Here's how the part is built. I have some questions about the finished solid (model axes, mm). Face numbers are marked on the shaded views. Round coordinates to 2 decimals unless told otherwise and drop trailing zeros. Loops run counter-clockwise (first coordinate to the right, second up) from the corner with the lowest first, then second, coordinate; pieces in that order, holes last. Notation, with made-up numbers: (32, 27) - (48, 27) arc R24 ccw to (48, 62) - close; hole circle Ø3 at (26.25, -30). An arc over 180 degrees is marked (long way). Answer as a JSON object with one key per item and string values. Group by question number.
1) I want a section at A-A, the plane y = 0. Please give me the cut outline in (x, z) (3 decimals).
2) Will these pins go through, and if not, where does the flat tip stop? P1, Ø4, axis at y = -2.5, z = 18.5, coming from the -X side; P2, Ø6, axis at x = -24.5, z = 106, coming from the -Y side; P3, Ø12, axis at y = -17.5, z = 15, coming from the -X side.
3) I want a section at B-B, the plane z = 23. Please give me the cut outline in (x, y) (3 decimals), then the cut area to 3 significant figures.
4) If we mould it in two halves opening along Y, with no side actions, what happens to the marked faces 1, 2 and 3? For each: pulls with the +Y half, pulls with the -Y half, needs draft (parallel to the pull), parting line crosses it, or undercut.
5) If I drill on line 1 along Y through (x, z) = (0, 42.5) (3 decimals); line 2 along Z through (x, y) = (-20.5, -23); line 3 along X through (y, z) = (-19, 71), over which ranges is the centre line in solid material (lowest first)? Write a range as [from, to].
from build123d import *

# Parameters (mm, degrees)
F0_R     = 38.1
F0_R_2   = 34.925
F1_DEPTH = 127
F2_R     = 34.925
F3_DEPTH = 2.54


# Not quite as in the source:
# - a fillet or chamfer that OpenCascade refuses, or shapes differently, is made with other operations: its cross-section is extruded or revolved along the edge and cut away or added


with BuildPart() as f1:
    # F0 (on Top) → F1 (new body)
    with BuildSketch(Plane.XY):
        Circle(F0_R)
        Circle(F0_R_2, mode=Mode.SUBTRACT)
    extrude(amount=F1_DEPTH)

    # F2 (on Top) → F3 (join)
    with BuildSketch(Plane.XY):
        Circle(F2_R)
    extrude(amount=F3_DEPTH)

    # F4: fillet of radius 5.08 on 1 edges, made by hand

    # F4_s1 → F4_t2 (revolve, cut)
    with BuildSketch(Plane.XZ):
        with BuildLine():
            ThreePointArc((38.1, 122.2907139607), (37.2321134838, 125.1305202921), (34.925, 127))
            Line((34.925, 127), (38.1, 127))
            Line((38.1, 127), (38.1, 122.2907139607))
        make_face()
    revolve(axis=Axis((0, 0, 127), (0, 0, 1)), mode=Mode.SUBTRACT)


solid = f1.part
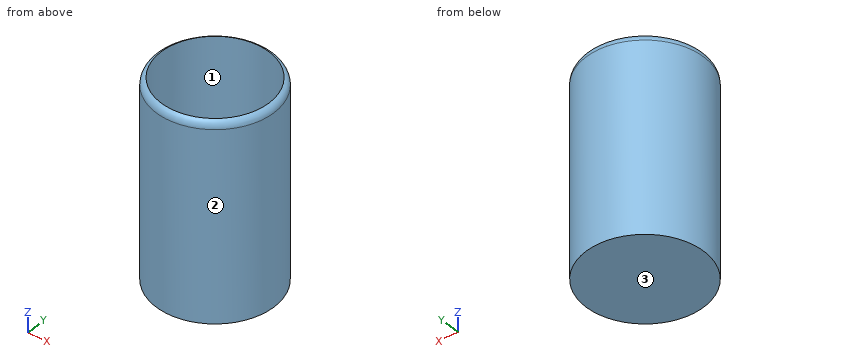
Outcome:
{
 "1": {"outline": "(-38.1, 0) - (38.1, 0) - (38.1, 122.291) arc R5.08 ccw to (34.925, 127) - (34.925, 2.54) - (-34.925, 2.54) - (-34.925, 127) arc R5.08 ccw to (-38.1, 122.291) - close"},
 "2": {"P1": "x = -38.1", "P2": "y = -31.45", "P3": "x = -36.32"},
 "3": {"outline": "circle Ø76.2 at (0, 0); hole circle Ø69.85 at (0, 0)", "area": "728 mm^2"},
 "4": {"face 1": "undercut", "face 2": "parting line crosses it", "face 3": "needs draft"},
 "5": {"line 1": "[-38.1, -34.925], [34.925, 38.1]", "line 2": "[0, 2.54]", "line 3": "[-33.02, -29.3], [29.3, 33.02]"}
}
